```python
from build123d import *

# Parameters (mm, degrees)
BOSS_EXTRUDE1_DEPTH     = 10
SKETCH2_W               = 2.9
SKETCH2_H               = 1
BOSS_EXTRUDE2_DEPTH     = 24
SKETCH3_R               = 1.5
CUT_EXTRUDE1_DEPTH      = 57.178287621
CUT_EXTRUDE2_DEPTH      = 56.452682697
CUT_EXTRUDE2_DEPTH_BACK = 56.452682697
SKETCH5_W               = 7
SKETCH5_H               = 35
FILLET1_START           = 1.5000001
FILLET1_DEPTH           = 10.4999999
FILLET1_START_2         = -12
FILLET1_2_DEPTH         = 10.499986243
FILLET1_START_3         = -1.500013757
FILLET1_3_DEPTH         = 3.000013857
FILLET1_4_OUTLINE_W     = 1.5
FILLET1_4_OUTLINE_H     = 6.418167134
SKETCH6_W               = 10
SKETCH6_H               = 9.539392014
CUT_EXTRUDE3_DEPTH      = 56.452682532
SKETCH7_R               = 1.5
CUT_EXTRUDE4_DEPTH      = 65.101043817


with BuildPart() as part:
    # Sketch1 → Boss-Extrude1 (new body)
    with BuildSketch(Plane.XY):
        with BuildLine():
            Line((-37.080992435, -15), (-12, -15))
            Line((-12, -15), (-12, 0))
            Line((-12, 0), (12, 0))
            Line((12, 0), (12, -15))
            Line((12, -15), (37.080992435, -15))
            ThreePointArc((37.080992435, -15), (0, -40), (-37.080992435, -15))
        make_face()
    extrude(amount=BOSS_EXTRUDE1_DEPTH)

    # Sketch2 → Boss-Extrude2 (add)
    with BuildSketch(Plane(origin=(12, 0, 0), x_dir=(0, 0, -1), z_dir=(1, 0, 0))):
        with Locations((-5, 0.5)):
            Rectangle(SKETCH2_W, SKETCH2_H)
    extrude(amount=-BOSS_EXTRUDE2_DEPTH)

    # Sketch3 → Cut-Extrude1 (cut, through all)
    with BuildSketch(Plane(origin=(0, 1, 0), x_dir=(1, 0, 0), z_dir=(0, 1, 0))):
        with Locations(Location((0, -5, 0), (0, 0, 270))):
            Circle(SKETCH3_R)
    extrude(amount=-CUT_EXTRUDE1_DEPTH, mode=Mode.SUBTRACT)

    # Sketch5 → Cut-Extrude2 (cut, two sides: drawn at the far end of the back side and taken through both)
    with BuildSketch(Plane(origin=(0, 0, 0), x_dir=(0, 0, -1), z_dir=(1, 0, 0)).offset(-CUT_EXTRUDE2_DEPTH_BACK)):
        with Locations((-3.5, -22.5)):
            Rectangle(SKETCH5_W, SKETCH5_H)
    extrude(amount=CUT_EXTRUDE2_DEPTH + CUT_EXTRUDE2_DEPTH_BACK, mode=Mode.SUBTRACT)

    # Fillet1: read off the stored shape, not the designer's step
    # Fillet1 outline → Fillet1 (add)
    with BuildSketch(Plane.YZ.offset(FILLET1_START)):
        with BuildLine():
            Line((-5, 7), (-14.539392014, 7))
            ThreePointArc((-14.539392014, 7), (-8.623312231, 5.062257748), (-5, 0))
            Line((-5, 0), (-5, 7))
        make_face()
    extrude(amount=FILLET1_DEPTH)

    # Fillet1 2 outline → Fillet1 2 (add)
    with BuildSketch(Plane.YZ.offset(FILLET1_START_2)):
        with BuildLine():
            Line((-5, 7), (-14.539392014, 7))
            ThreePointArc((-14.539392014, 7), (-8.623312231, 5.062257748), (-5, 0))
            Line((-5, 0), (-5, 7))
        make_face()
    extrude(amount=FILLET1_2_DEPTH)

    # Fillet1 3 outline → Fillet1 3 (add)
    with BuildSketch(Plane.YZ.offset(FILLET1_START_3)):
        with BuildLine():
            Line((-5, 7), (-14.539392014, 7))
            ThreePointArc((-14.539392014, 7), (-8.623312231, 5.062257748), (-5, 0))
            Line((-5, 0), (-5, 7))
        make_face()
    extrude(amount=FILLET1_3_DEPTH)

    # Fillet1 4 outline → Fillet1 4 (revolve, cut)
    with BuildSketch(Plane.XY.offset(5)):
        with Locations((0.75, -8.209083567)):
            Rectangle(FILLET1_4_OUTLINE_W, FILLET1_4_OUTLINE_H)
    revolve(axis=Axis((0, 0, 5), (0, 1, 0)), mode=Mode.SUBTRACT)

    # Sketch6 → Cut-Extrude3 (cut, through all)
    with BuildSketch(Plane(origin=(0, 0, 0), x_dir=(-1, 0, 0), z_dir=(0, 0, -1))):
        with Locations((0, -9.769696007)):
            Rectangle(SKETCH6_W, SKETCH6_H)
    extrude(amount=-CUT_EXTRUDE3_DEPTH, mode=Mode.SUBTRACT)

    # Sketch7 → Cut-Extrude4 (cut, through all)
    with BuildSketch(Plane.ZY.offset(12)):
        with Locations((5, -3)):
            Circle(SKETCH7_R)
    extrude(amount=-CUT_EXTRUDE4_DEPTH, mode=Mode.SUBTRACT)


solid = part.part
```
Verification items for the finished model (mm, model axes). A direction names the side the tool comes from. Round coordinates to 2 decimals unless told otherwise and drop trailing zeros. Write each loop counter-clockwise with the first axis right and the second up, starting at its lowest first coordinate (ties: lowest second). Pieces come first, ordered by that corner, then holes. Notation, with made-up numbers: (-1.75, 68.25) - (39.25, 68.25) arc R18 cw to (39.25, 75.25) - close; hole circle Ø5 at (23, 64). An arc over 180 degrees is marked (long way). Answer as a JSON object with one key per item and string values. Group by question number.
Q1. Tool access check on faces 1 (the flat face through (0, 0, 8)), 2 (the flat face through (-12, -5, 6)), 3 (the flat face through (24, -15, 8)), 4 (the flat face through (5, -9, 7)). Record the directions out of +Z, -Z, +X, -X, +Y, -Y that give a thin tool (end or side, any length) a straight path to the whole face; none if there is none.
Q2. Section check D-D, the plane y = -20. Enter the section's corners in (x, z).
Q3. Mould release check, pull along Y, two halves, no side actions. Record for faces 5 (the flat face through (1.2, -5, 3.8)), 6 (the flat face through (-25, -15, 8)), 7 (the cylindrical face through (8.45, -8.69, 5.11)): released by +Y, released by -Y, zero draft, split by the parting line, or undercut.
Q4. Thickness scan on line 1 (Z direction, x = -3, y = -3); line 2 (Y direction, x = -0.5, z = 9.75); line 3 (X direction, y = -7, z = 9.5). Record the ranges inside material, lowest first.
Q5. Go/stop test with flat-tipped pins: pin 1 Ø0.9 at (x, z) = (1, 9) entering from +Y; pin 2 Ø4 at (y, z) = (-26.5, 6) entering from +X; pin 3 Ø5 at (x, y) = (-13, -17) entering from -Z; pin 4 Ø1.8 at (x, z) = (0, 5) entering from -Y. Record where each tip stops, or that it passes through.
Q6. Section check B-B, the plane z = 5. Enter the section's corners in (x, y), plus the area to 3 significant figures.
Q7. Section check C-C, the plane z = 1. Enter the section's corners in (x, y), plus the area to 3 significant figures.
Q8. Section check A-A, the plane x = 11. Enter the section's corners in (y, z), plus the area to 3 significant figures.
Found:
{
 "1": {"face 1": "+Z, +X, -X, +Y", "face 2": "+Z, -Z, -X, +Y", "face 3": "+Z, -Z, +X, +Y", "face 4": "+Z, -Z"},
 "2": {"outline": "(-34.64, 7) - (34.64, 7) - (34.64, 10) - (-34.64, 10) - close"},
 "3": {"face 5": "undercut", "face 6": "released by +Y", "face 7": "released by -Y"},
 "4": {"line 1": "z = 0 to 3.5, 6.5 to 10", "line 2": "y = -40 to -14.54, -5 to 0", "line 3": "x = -12 to -5, 5 to 12"},
 "5": {"pin 1": "stops at y = 0", "pin 2": "stops at x = 31.41", "pin 3": "stops at z = 7", "pin 4": "passes through"},
 "6": {"outline": "(-12, -8.54) - (-5, -8.54) - (-5, -5) - (-1.5, -5) - (-1.5, -4.5) - (-12, -4.5) - close; (-12, -1.5) - (-1.5, -1.5) - (-1.5, 1) - (-12, 1) - close; (1.5, -5) - (5, -5) - (5, -8.54) - (12, -8.54) - (12, -4.5) - (1.5, -4.5) - close; (1.5, -1.5) - (12, -1.5) - (12, 1) - (1.5, 1) - close", "area": "113 mm^2"},
 "7": {"outline": "(-12, -5.37) - (-5, -5.37) - (-5, -5) - (5, -5) - (5, -5.37) - (12, -5.37) - (12, 0) - (-12, 0) - close", "area": "125 mm^2"},
 "8": {"outline": "(-38.46, 7) - (-14.54, 7) arc R10 cw to (-5, 0) - (0, 0) - (0, 3.55) - (1, 3.55) - (1, 6.45) - (0, 6.45) - (0, 10) - (-38.46, 10) - close; hole circle Ø3 at (-3, 5)", "area": "164 mm^2"}
}
